Part print with two shaded views. Sizes in mm from the minimum x, y, z corner. Round coordinates to 2 decimals unless told otherwise and drop trailing zeros. Write each loop counter-clockwise with the first axis right and the second up, starting at its lowest first coordinate (ties: lowest second). Pieces come first, ordered by that corner, then holes. Notation, with made-up numbers: (84, -32.5) -> (96, -32.5) arc R30 ccw to (96, -10.5) -> close; hole circle Ø6 at (43, 46.5). An arc over 180 degrees is marked (long way). Return JSON: item names as keys, results as strings.
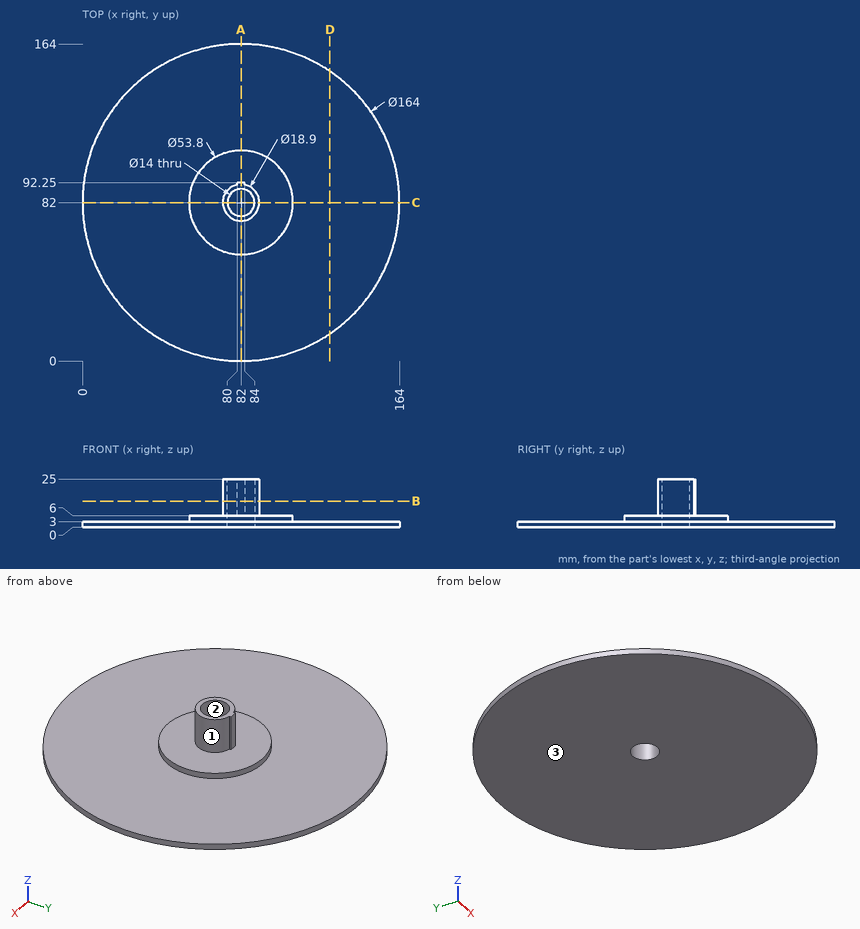
Q1. Saw through at B-B on z = 13.5. List the corners of the cut face in (x, y), then the cut area to 3 significant figures.
Verdict:
{"outline": "(80, 91.24) arc R9.45 ccw (long way) to (84, 91.24) -> (84, 92.25) -> (80, 92.25) -> close; hole circle Ø14 at (82, 82)", "area": "130 mm²"}
Q2. Wall check: L1, parallel to Y at x = 82, z = 17.75; L2, parallel to Y at x = 82, z = 5; L3, parallel to Z at x = 148, y = 94. Give the ranges that are in metal, low to high.
Verdict:
{"L1": "y = 72.55 to 75, 89 to 92.25", "L2": "y = 55.1 to 75, 89 to 108.9", "L3": "z = 0 to 3"}
Q3. Saw through at C-C on y = 82. List the corners of the cut face in (x, z), then the cut area to 4 significant figures.
Verdict:
{"outline": "(0, 0) -> (75, 0) -> (75, 25) -> (72.55, 25) -> (72.55, 6) -> (55.1, 6) -> (55.1, 3) -> (0, 3) -> close; (89, 0) -> (164, 0) -> (164, 3) -> (108.9, 3) -> (108.9, 6) -> (91.45, 6) -> (91.45, 25) -> (89, 25) -> close", "area": "662.5 mm²"}
Q4. Saw through at D-D on x = 128. List the corners of the cut face in (y, z).
Verdict:
{"outline": "(14.12, 0) -> (149.88, 0) -> (149.88, 3) -> (14.12, 3) -> close"}
Q5. Pin check, flat tips, straight feed: pin 1 Ø12 at (x, y) = (102, 40.5) entering from +Z; pin 2 Ø4 at (x, z) = (81.5, 9.5) entering from +Y; pin 3 Ø11 at (x, y) = (82, 82) entering from +Z; pin 4 Ø8 at (x, z) = (68, 5) entering from -Y. Stop position of each tip, or through.
Verdict:
{"pin 1": "stops at z = 3", "pin 2": "stops at y = 92.25", "pin 3": "passes through", "pin 4": "stops at y = 0.68"}
Q6. Two-plate mould, pull along X, no slides. Class the marked faces 1, 2 and 3: +X half, -X half, draft (parallel to the pull), parting line (faces both ways), or undercut.
Verdict:
{"face 1": "parting line", "face 2": "undercut", "face 3": "draft"}
Q7. Saw through at A-A on x = 82. List the corners of the cut face in (y, z).
Verdict:
{"outline": "(0, 0) -> (75, 0) -> (75, 25) -> (72.55, 25) -> (72.55, 6) -> (55.1, 6) -> (55.1, 3) -> (0, 3) -> close; (89, 0) -> (164, 0) -> (164, 3) -> (108.9, 3) -> (108.9, 6) -> (92.25, 6) -> (92.25, 25) -> (89, 25) -> close"}
